Work out the finished part from the listing and answer in its coordinate system (mm). A direction names the side the tool comes from. Give positions to 0.01 mm unless a question says otherwise; leave off trailing zeros. Order: outer loops, then holes, each group sorted by start corner. A loop starts at its lowest first (then second) coordinate and runs counter-clockwise, first axis right, second up. Notation, with made-up numbers: (4, 33.5) - (60, 33.5) arc R30 ccw to (60, 56.5) - close; hole circle Ø3 at (26.25, 38). An arc over 180 degrees is marked (long way). Put each result on its own line as item: value.
```python
from build123d import *

# Parameters (mm, degrees)
SKETCH_1_R            = 3
EXTRUDE_251_DEPTH     = 2.5
CHAMFER_1_SIZE        = 1.5
CUT_EXTRUDE_459_DEPTH = 1.3
SKETCH_3_R            = 1.5
EXTRUDE_571_DEPTH     = 35


with BuildPart() as part:
    # 草图1 → Extrude 251 (new body)
    with BuildSketch(Plane(origin=(0, 0, 0), x_dir=(1, 0, 0), z_dir=(0, 1, 0))):
        Circle(SKETCH_1_R)
    extrude(amount=EXTRUDE_251_DEPTH)

    # 倒角1
    chamfer_1_edges = [part.edges().sort_by_distance(p)[0] for p in [
        (-3, 0, 0),
    ]]
    chamfer(chamfer_1_edges, length=CHAMFER_1_SIZE)

    # 草图2 → Cut-Extrude 459 (cut)
    with BuildSketch(Plane(origin=(0, 2.5, 0), x_dir=(1, 0, 0), z_dir=(0, 1, 0))):
        Polygon((1.443375673, 0), (0.721687836, 1.25), (-0.721687836, 1.25), (-1.443375673, 0), (-0.721687836, -1.25), (0.721687836, -1.25), align=None)
    extrude(amount=-CUT_EXTRUDE_459_DEPTH, mode=Mode.SUBTRACT)

    # 草图3 → Extrude 571 (add)
    with BuildSketch(Plane.XZ):
        Circle(SKETCH_3_R)
    extrude(amount=EXTRUDE_571_DEPTH)


solid = part.part
```
(1) Determine the mould class of faces 1 (the face through (1.3, 2.5, 0.6)), 2 (the face through (1.08, 1.86, 0.63)), 3 (the face through (-1.5, -17.26, 0.07)) for opening direction X: pulls with the +X half, pulls with the -X half, needs draft (parallel to the pull), parting line crosses it, or undercut.
Geometry check:
face 1: needs draft
face 2: undercut
face 3: parting line crosses it
(2) Section A-A, the plane x = 0 is taken. Write down the section's boundary in (y, z).
Geometry check:
outline: (-35, -1.5) - (0, -1.5) - (1.5, -3) - (2.5, -3) - (2.5, -1.25) - (1.2, -1.25) - (1.2, 1.25) - (2.5, 1.25) - (2.5, 3) - (1.5, 3) - (0, 1.5) - (-35, 1.5) - close
(3) Straight lines are drawn through the part: line 1 (Y direction, x = -0.2, z = 0.45); line 2 (X direction, y = -24.5, z = -0.6); line 3 (Y direction, x = -1.1, z = -1.25). For each, find the intervals that lie inside material, in ascending order.
Geometry check:
line 1: y = -35 to 1.2
line 2: x = -1.37 to 1.37
line 3: y = 0.17 to 2.5
(4) Section B-B, the plane y = -25 is taken. Write down the section's boundary in (x, z), then the cut area to 3 significant figures.
Geometry check:
outline: circle Ø3 at (0, 0)
area: 7.07 mm²
(5) Given pin 1 (2 mm diameter, centred on y = -7, z = 1, fed in from -X); pin 2 (1.5 mm diameter, centred on x = -0.5, y = -13, fed in from -Z); pin 3 (0.8 mm diameter, centred on x = 0, z = -0.5, fed in from +Y), each flat-ended and moving along its own axis, determine where each tip first touches the part or whether it passes through.
Geometry check:
pin 1: stops at x = -1.5
pin 2: stops at z = -1.5
pin 3: stops at y = 1.2
(6) A tool of negligible diameter and unlimited length cuts with its end or side. For faces 4 (the face through (0, 2, 1.25)), 5 (the face through (0, -35, 0)), from which of +Z, -Z, +X, -X, +Y, -Y can it reach the whole face along a straight path? Write none if from no direction.
Geometry check:
face 4: +Y
face 5: +Z, -Z, +X, -X, -Y
